Solid Edge part; units mm, degrees
sketch "Sketch1" plane through (0, 0, 0) normal (0, 0, 1) x (1, 0, 0)
  line L0 (-3.175, -3.175) -> (3.175, -3.175)
  line L1 (3.175, -3.175) -> (3.175, 3.175)
  line L2 (3.175, 3.175) -> (-3.175, 3.175)
  line L3 (-3.175, 3.175) -> (-3.175, -3.175)
  dimension "D1" = 3.175
  dimension "D2" = 3.175
extrude "Protrusion1" add sketch "Sketch1" along normal blind 127
sketch "Sketch2" plane through (0, 0, 0) normal (0, 0, -1) x (1, 0, 0)
  line L0 (-3.175, -3.175) -> (-3.175, 3.175)
  line L1 (-41.6698, -63.5) -> (-36.1706, -60.325)
  arc A0 (-3.175, -3.175) -> (-36.1706, -60.325) centre (-3.175, -41.275) ccw
  arc A1 (-41.6698, -63.5) -> (-3.175, 3.175) centre (-3.175, -41.275) cw
extrude "ExtrudedProtrusion_2" add sketch "Sketch2" against normal blind 127
mirror "Mirror1" about plane through (0, 0, 0) normal (1, 0, 0) of "ExtrudedProtrusion_2"
properties part number "SPaRC - 02 - 004"
The listing builds one solid part. Answer for the finished solid, in the listing's coordinates (mm). A direction names the side the tool comes from. Coordinates: 2 decimals unless noted, no trailing zeros. Write each loop counter-clockwise with the first axis right and the second up, starting at its lowest first coordinate (ties: lowest second). Pieces come first, ordered by that corner, then holes. Notation, with made-up numbers: M 72.25,6 L 125.25,6 A25 cw 125.25,20 Z; hole C 43.5,20.25 d9. An arc over 180 degrees is marked long. Put each result on its own line as item: value. Start each with the question number.
1. A cutting plane is placed at A-A on z = 22.5. Write down the section's boundary in (x, y) (3 decimals), then the cut area to 3 significant figures.
2. A cutting plane is placed at C-C on x = 39.5. Write down the section's boundary in (y, z).
3. Consider line 1 (X direction, y = 31.5, z = 77); line 2 (X direction, y = 23.5, z = 118.5); line 3 (X direction, y = 2, z = 80). Determine where each line is inside the solid, lowest interval first. Write a range as from..to.
4. A cutting plane is placed at D-D on x = 1. Write down the section's boundary in (y, z) (3 decimals).
5. A cutting plane is placed at B-B on y = 13.5. Write down the section's boundary in (x, z).
6. For a pull along X with two mould halves and no side action, classify faces 4 (the flat face through (0, 3.175, 63)), 5 (the flat face through (-38.959, 61.935, 62.611)), 6 (the cylindrical face through (41.992, 19.617, 62.611)), 7 (the cylindrical face through (-41.34, 18.49, 62.61)) as pulls with the +X half, pulls with the -X half, needs draft (parallel to the pull), parting line crosses it, or undercut.
7. Which of the six approach directions +Z, -Z, +X, -X, +Y, -Y give full straight-line access (tool end or side, diameter ignored) to faces 1 (the flat face through (38.9, 61.9, 62.6)), 2 (the cylindrical face through (36.446, 22.711, 62.611)), 3 (the flat face through (0, 3, 0))?
8. Flat-ended cylindrical pins translate along their axes: P1, Ø3, axis at x = 0, z = 39, coming from the +Y side (3 decimals); P2, Ø2, axis at y = 28.5, z = 75.5, coming from the -X side; P3, Ø10, axis at y = 8.5, z = 85, coming from the +X side. Find the tip coordinate at first contact, or state that the pin passes through.
Resolved:
1. outline: M -41.67,63.5 A44.45 ccw -3.175,-3.175 L 3.175,-3.175 A44.45 ccw 41.67,63.5 L 36.171,60.325 A38.1 cw 3.175,3.175 L -3.175,3.175 A38.1 cw -36.171,60.325 Z
1. area: 1,140 mm2
2. outline: M 15.66,0 L 29.78,0 L 29.78,127 L 15.66,127 Z; M 52.77,0 L 62.25,0 L 62.25,127 L 52.77,127 Z
3. line 1: x = -46.54..-40, 40..46.54
3. line 2: x = -43.92..-36.87, 36.87..43.92
3. line 3: x = -23.99..23.99
4. outline: M -3.175,0 L 3.175,0 L 3.175,127 L -3.175,127 Z
5. outline: M -37.88,0 L -29.25,0 L -29.25,127 L -37.88,127 Z; M 29.25,0 L 37.88,0 L 37.88,127 L 29.25,127 Z
6. face 4: undercut
6. face 5: undercut
6. face 6: pulls with the +X half
6. face 7: pulls with the -X half
7. face 1: +Z, -Z, +Y
7. face 2: +Z, -Z
7. face 3: -Z, +X, -X, +Y, -Y
8. P1: stops at y = 3.175
8. P2: stops at x = -46.04
8. P3: stops at x = 37.88
